```python
from build123d import *

# Parameters (mm, degrees)
F0_R      = 30
F2_R      = 6
F4_R      = 25
F5_R      = 4
F7_R      = 6
F7_R_2    = 4
F8_DEPTH  = 10
F9_R      = 3
F9_R_2    = 27
F10_DEPTH = 1


with BuildPart() as f3:
    # F0 (on Top) → F3 section 0
    with BuildSketch(Plane.XY):
        Circle(F0_R)
    # F2 (on offset) → F3 section 1
    with BuildSketch(Plane.XY.offset(30)):
        Circle(F2_R)
    loft()

    # F4 (on Top) → F6 section 0
    with BuildSketch(Plane.XY):
        Circle(F4_R)
    # F5 (on offset) → F6 section 1
    with BuildSketch(Plane.XY.offset(30)):
        Circle(F5_R)
    loft(mode=Mode.SUBTRACT)

    # F7 (on face) → F8 (join)
    with BuildSketch(Plane.XY.offset(30)):
        Circle(F7_R)
        Circle(F7_R_2, mode=Mode.SUBTRACT)
    extrude(amount=F8_DEPTH)

    # F9 (on Top) → F10 (join)
    with BuildSketch(Plane.XY):
        with BuildLine():
            ThreePointArc((6, -35.496479), (0, 36), (-6, -35.496479))
            Line((-6, -35.496479), (-6, -41.393877))
            ThreePointArc((-6, -41.393877), (0, -47.393877), (6, -41.393877))
            Line((6, -41.393877), (6, -35.496479))
        make_face()
        with Locations((0, -41.393877)):
            Circle(F9_R, mode=Mode.SUBTRACT)
        Circle(F9_R_2, mode=Mode.SUBTRACT)
    extrude(amount=F10_DEPTH)


solid = f3.part
```
Work out the finished part from the listing and answer in its coordinate system (mm). A direction names the side the tool comes from. Give positions to 0.01 mm unless a question says otherwise; leave off trailing zeros. Loops run counter-clockwise (first coordinate to the right, second up) from the corner with the lowest first, then second, coordinate; pieces in that order, holes last. Notation, with made-up numbers: (14.25, 21) -> (23.25, 21) arc R13 ccw to (23.25, 33) -> close; hole circle Ø11 at (43.25, 21.25). An arc over 180 degrees is marked (long way). Write item = value, one per line. Start each with the question number.
(1) Which of the six approach directions +Z, -Z, +X, -X, +Y, -Y give full straight-line access (tool end or side, diameter ignored) to faces 1 (the flat face through (0, -30, 1)), 2 (the cylindrical face through (-0.132, -47.392, 0.493))?
(2) The mould has two halves that part along X. Classify faces 3 (the cylindrical face through (-0.65, -44.323, 0.493)), 4 (the conical face through (9.26, 2.91, 25.37)), 5 (the flat face through (-1.42, -3.92, 40)): +X half, -X half, draft (parallel to the pull), parting line (faces both ways), or undercut.
(3) Find the intervals of material crossed by probe 1 along Y at (x, z) = (0, 32); probe 2 along Y at (x, z) = (0, 0.55) (3 decimals); probe 3 along Z at (x, y) = (2, 31), in increasing order. Write a range as from..to.
(4) Find section C-C on z = 19. Give the vertices of the cut face in (x, y).
(5) Find section A-A on x = 0. Give the vertices of the cut face in (y, z), and give its area (3 significant figures).
(6) Given pin 1 Ø0.5 at (y, z) = (-39.5, 0.5) entering from +X; pin 2 Ø10 at (x, y) = (-22, -36.5) entering from -Z; pin 3 Ø1 at (x, y) = (5.5, -20) entering from +Z; pin 4 Ø3 at (x, y) = (-5, -10) entering from -Z, each flat-ended and moving along its own axis, determine where each tip first touches the part or whether it passes through.
(7) Find section B-B on z = 10. Give the vertices of the cut face in (x, y), and give its area (3 significant figures).
From the geometry:
q1.face_1 = +Z
q1.face_2 = +Z, -Z, -Y
q2.face_3 = undercut
q2.face_4 = parting line
q2.face_5 = draft
q3.probe_1 = -6..-4, 4..6
q3.probe_2 = -47.394..-44.394, -38.394..-24.615, 24.615..36
q3.probe_3 = 0..1
q4.outline = circle Ø29.6 at (0, 0); hole circle Ø23.4 at (0, 0)
q5.outline = (-47.39, 0) -> (-44.39, 0) -> (-44.39, 1) -> (-47.39, 1) -> close; (-38.39, 0) -> (-25, 0) -> (-4, 30) -> (-4, 40) -> (-6, 40) -> (-6, 30) -> (-29.2, 1) -> (-38.39, 1) -> close; (4, 30) -> (25, 0) -> (36, 0) -> (36, 1) -> (29.2, 1) -> (6, 30) -> (6, 40) -> (4, 40) -> close
q5.area = 268 mm^2
q6.pin_1 = 6
q6.pin_2 = through
q6.pin_3 = 12.2
q6.pin_4 = 17.6
q7.outline = circle Ø44 at (0, 0); hole circle Ø36 at (0, 0)
q7.area = 503 mm^2
